Check sheet for the modelled part. Datum: model origin and axes. Units: mm. Face numbers are marked on the shaded views. A direction names the side the tool comes from. Give positions to 0.01 mm unless a question says otherwise; leave off trailing zeros. Write each loop counter-clockwise with the first axis right and the second up, starting at its lowest first coordinate (ties: lowest second). Pieces come first, ordered by that corner, then holes. Notation, with made-up numbers: M -24,-2 L 5,-2 A22 cw 5,9 Z; hole C 8,-39.5 d10. An arc over 180 degrees is marked long. Write item = value, one per line. Start each with the question number.
1) Sectioned sample at D-D, the plane y = 11.25. Record the cut outline in (x, z).
2) Gauge pin test, flat ends, axial feed: pin 1 (0.6 mm diameter, centred on y = 7.5, z = 23, fed in from +X); pin 2 (7 mm diameter, centred on x = 25.5, y = 5.5, fed in from +Z); pin 3 (7 mm diameter, centred on y = 10, z = -5, fed in from -X). Record the tip position at first contact, or that the pin passes through.
3) Sectioned sample at B-B, the plane x = 10. Record the cut outline in (y, z).
4) Sectioned sample at A-A, the plane z = -19. Record the cut outline in (x, y), then the cut area to 3 significant figures.
5) Scan lines: L1, parallel to Z at x = 11, y = 11; L2, parallel to Y at x = 36, z = -19; L3, parallel to Z at x = 2, y = 11.5. Record each from-to range of solid material in increasing order.
6) Set-up check for the marked faces 1, 2 and 3: record each of +Z, -Z, +X, -X, +Y, -Y from which the full face is reachable in a straight line by a thin tool's end or side.
7) Draft check along X on the marked faces 4, 5, 6 and 7. Enter one of: pulls with the +X half, pulls with the -X half, needs draft (parallel to the pull), parting line crosses it, or undercut.
8) Sectioned sample at C-C, the plane x = 28. Record the cut outline in (y, z), then the cut area to 3 significant figures.
Autodesk Inventor part; units mm, degrees
ref_plane "YZ Plane" through (0, 0, 0) normal (1, 0, 0) x (0, 1, 0)
ref_plane "XZ Plane" through (0, 0, 0) normal (0, 1, 0) x (-1, 0, 0)
ref_plane "XY Plane" through (0, 0, 0) normal (0, 0, 1) x (1, 0, 0)
sketch "Skizze1" plane through (0, 0, 0) normal (0, 1, 0) x (-1, 0, 0)
  line L0 (0, -22) -> (0, -27)
  line L1 (0, -27) -> (-40, -27)
  line L2 (-40, -27) -> (-40, 4)
  line L3 (-17, 27) -> (0, 27)
  line L4 (0, 27) -> (0, 22)
  line L5 (0, -22) -> (-3, -22)
  line L6 (-3, -22) -> (-3, -25)
  line L7 (-3, -25) -> (-17, -25)
  line L8 (-17, -25) -> (-17, -22)
  line L9 (-17, -22) -> (-35, -22)
  line L10 (-35, -22) -> (-35, 4)
  line L11 (-17, 24) -> (-17, 24)
  line L12 (-17, 24) -> (-3, 24)
  line L13 (-3, 24) -> (-3, 22)
  line L14 (-3, 22) -> (0, 22)
  line L15 (0, 0) -> (-33.6444, 0) construction
  arc A0 (-33.5355, 7.5355) -> (-35, 4) centre (-30, 4) ccw
  line L16 (-33.5355, 7.5355) -> (-19.0711, 22)
  line L17 (-19.0711, 22) -> (-17, 22)
  line L18 (-17, 22) -> (-17, 24)
  line L19 (-17, 24) -> (-17, 24)
  arc A1 (-38.5355, 7.5355) -> (-40, 4) centre (-35, 4) ccw
  line L20 (-38.5355, 7.5355) -> (-20.5355, 25.5355)
  arc A2 (-17, 27) -> (-20.5355, 25.5355) centre (-17, 22) ccw
  point P0 (-1.5, 22)
  dimension "d2" = 5
  dimension "d3" = 40
  dimension "d4" = 3
  dimension "d5" = 14
  dimension "d6" = 54
  dimension "d7" = 3
  dimension "d8" = 2
  dimension "d12" = 26
  dimension "d16" = 2
  dimension "d17" = 3
  dimension "d18" = 5
  dimension "d19" = 5
  dimension "d20" = 5
  dimension "d21" = 45
extrude "Extrusion1" add sketch "Skizze1" along normal blind 14
fillet "Rundung1" radius 2 3 edges at (0, 7, -27) (40, 7, -27) (0, 7, 27)
fillet "Rundung2" radius 0.2 1 edges at (35, 7, -22)
sketch "Skizze2" plane through (35, 0, 4) normal (-1, 0, 0) x (0, 0, 1)
  line L0 (-31, 14) -> (-31, 0)
  point P0 (-4, 0)
  point P1 (-23, 7)
  point P2 (-4, 7)
  point P3 (-31, 7)
  dimension "d26" = 19
  dimension "d27" = 8
hole "Bohrung1" at (35, 7, -19) at (35, 7, 0) direction (1, 0, 0) diameter 4.134 depth 5
sketch "Skizze3" plane through (3, 0, -25) normal (0, 0, 1) x (1, 0, 0)
  line L0 (-3, 14) -> (-1, 14)
  line L1 (-1, 14) -> (-1, 0)
  line L2 (-1, 0) -> (-3, 0)
  line L3 (-3, 0) -> (-3, 14)
  point P0 (-3, 0)
  point P1 (7, 7)
  point P2 (-3, 7)
  dimension "d42" = 10
hole "Bohrung2" at (10, 7, -25) direction (0, 0, -1) diameter 4 end through all
sketch "Skizze5" plane through (17, 0, 24) normal (0, 0, -1) x (-1, 0, 0)
  line L0 (17, 14) -> (17, 0)
  point P0 (7, 7)
  point P1 (17, 7)
  dimension "d44" = 10
hole "Bohrung3" at (10, 7, 24) direction (0, 0, 1) diameter 4 end through all
properties part number "114"
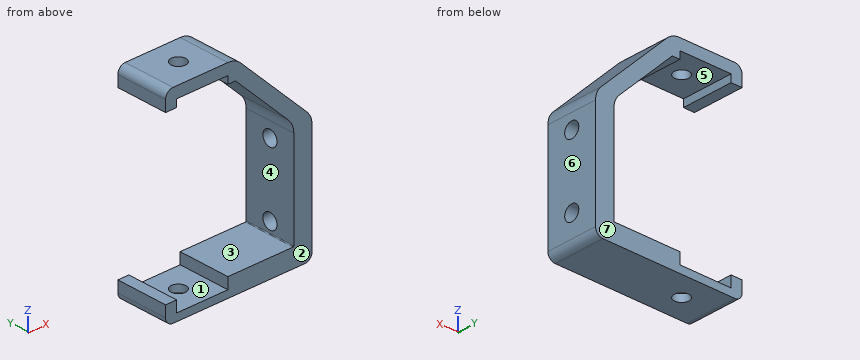
Data:
q1.outline = M 0,-25 A2 ccw 2,-27 L 38,-27 A2 ccw 40,-25 L 40,4 A5 ccw 38.54,7.54 L 20.54,25.54 A5 ccw 17,27 L 2,27 A2 ccw 0,25 L 0,22 L 3,22 L 3,24 L 17,24 L 17,22 L 19.07,22 L 33.54,7.54 A5 cw 35,4 L 35,-21.8 A0.2 cw 34.8,-22 L 17,-22 L 17,-25 L 3,-25 L 3,-22 L 0,-22 Z
q2.pin_1 = 23.37
q2.pin_2 = 24.07
q2.pin_3 = 35
q3.outline = M 0,-27 L 5,-27 L 5,-25 L 0,-25 Z; M 0,24 L 5,24 L 5,27 L 0,27 Z; M 9,-27 L 14,-27 L 14,-25 L 9,-25 Z; M 9,24 L 14,24 L 14,27 L 9,27 Z
q4.outline = M 35,0 L 40,0 L 40,4.93 L 35,4.93 Z; M 35,9.07 L 40,9.07 L 40,14 L 35,14 Z
q4.area = 49.3 mm2
q5.L1 = -27 to -25, 24 to 27
q5.L2 = 0 to 4.93, 9.07 to 14
q5.L3 = -27 to -22, 22 to 27
q6.face_1 = +Y, -Y
q6.face_2 = +Z, -Z, +X, -X, -Y
q6.face_3 = -X, +Y, -Y
q7.face_4 = pulls with the -X half
q7.face_5 = undercut
q7.face_6 = pulls with the +X half
q7.face_7 = needs draft
q8.outline = M 0,-27 L 14,-27 L 14,-22 L 0,-22 Z; M 0,13.07 L 14,13.07 L 14,18.07 L 0,18.07 Z
q8.area = 140 mm2
